Geometry check sheet. Reference: the model listing, model coordinates, mm. Coordinates: 2 decimals unless noted, no trailing zeros. Write each loop counter-clockwise with the first axis right and the second up, starting at its lowest first coordinate (ties: lowest second). Pieces come first, ordered by that corner, then holes. Notation, with made-up numbers: (54.25, 28.5) -> (68.25, 28.5) arc R21 cw to (68.25, 51.5) -> close; hole circle Ø6 at (-14.5, 27.5). An arc over 180 degrees is marked (long way). One line per question, with ' | ' between items.
```python
from build123d import *

# Parameters (mm, degrees)
F1_DEPTH = 6.8
F2_SIZE  = 2.54
F3_SIZE  = 0.508
F5_DEPTH = 6.801


with BuildPart() as f1:
    # F0 (on Top) → F1 (new body)
    with BuildSketch(Plane.XY):
        with BuildLine():
            ThreePointArc((0, -11.175), (-7.9019182798, -7.9019182798), (-11.175, 0))
            Line((-11.175, 0), (-19.135426009, 0))
            ThreePointArc((-19.135426009, 0), (-13.5307894918, -13.5307894918), (0, -19.135426009))
            Line((0, -19.135426009), (0, -11.175))
        make_face()
        with BuildLine():
            Line((-19.135426009, 0), (-11.175, 0))
            ThreePointArc((-11.175, 0), (-10.3243537758, 4.2764873567), (-7.9019182798, 7.9019182798))
            Line((-7.9019182798, 7.9019182798), (-10.1350344611, 10.1350344611))
            ThreePointArc((-10.1350344611, 10.1350344611), (-13.6801442317, 7.7438710244), (-17.8637937449, 6.8592566349))
            ThreePointArc((-17.8637937449, 6.8592566349), (-18.8148323403, 3.4880671653), (-19.135426009, 0))
        make_face()
        with BuildLine():
            ThreePointArc((-7.9019182798, 7.9019182798), (-4.2764873567, 10.3243537758), (0, 11.175))
            Line((0, 11.175), (0, 19.135426009))
            ThreePointArc((0, 19.135426009), (-3.4923449173, 18.8140387882), (-6.8673791432, 17.8606727826))
            ThreePointArc((-6.8673791432, 17.8606727826), (-7.7488210815, 13.6796226746), (-10.1350344611, 10.1350344611))
            Line((-10.1350344611, 10.1350344611), (-7.9019182798, 7.9019182798))
        make_face()
        with BuildLine():
            Line((0, 19.135426009), (0, 11.175))
            ThreePointArc((0, 11.175), (7.9019182798, 7.9019182798), (11.175, 0))
            Line((11.175, 0), (19.135426009, 0))
            ThreePointArc((19.135426009, 0), (13.5307894918, 13.5307894918), (0, 19.135426009))
        make_face()
        with BuildLine():
            Line((19.135426009, 0), (11.175, 0))
            ThreePointArc((11.175, 0), (10.3243537758, -4.2764873567), (7.9019182798, -7.9019182798))
            Line((7.9019182798, -7.9019182798), (10.139134376, -10.139134376))
            ThreePointArc((10.139134376, -10.139134376), (13.6813541851, -7.7515602366), (17.8606227185, -6.8675093486))
            ThreePointArc((17.8606227185, -6.8675093486), (18.8140260583, -3.4924134951), (19.135426009, 0))
        make_face()
        with BuildLine():
            ThreePointArc((7.9019182798, -7.9019182798), (4.2764873567, -10.3243537758), (0, -11.175))
            Line((0, -11.175), (0, -19.135426009))
            ThreePointArc((0, -19.135426009), (3.4924134951, -18.8140260583), (6.8675093486, -17.8606227185))
            ThreePointArc((6.8675093486, -17.8606227185), (7.7515602366, -13.6813541851), (10.139134376, -10.139134376))
            Line((10.139134376, -10.139134376), (7.9019182798, -7.9019182798))
        make_face()
        with BuildLine():
            Line((-36.0821053116, 0), (-19.135426009, 0))
            ThreePointArc((-19.135426009, 0), (-18.8148323403, 3.4880671653), (-17.8637937449, 6.8592566349))
            ThreePointArc((-17.8637937449, 6.8592566349), (-22.2382076575, 7.6759923472), (-25.9470708504, 10.1350344611))
            Line((-25.9470708504, 10.1350344611), (-36.0821053116, 0))
        make_face()
        with BuildLine():
            ThreePointArc((-6.8673791432, 17.8606727826), (-3.4923449173, 18.8140387882), (0, 19.135426009))
            Line((0, 19.135426009), (0, 36.0821053116))
            Line((0, 36.0821053116), (-10.1432364193, 25.9388688923))
            ThreePointArc((-10.1432364193, 25.9388688923), (-7.7178089445, 22.3120170041), (-6.8660526558, 18.0328506976))
            ThreePointArc((-6.8660526558, 18.0328506976), (-6.8663842826, 17.9467591853), (-6.8673791432, 17.8606727826))
        make_face()
        with BuildLine():
            Line((36.0821053116, 0), (19.135426009, 0))
            ThreePointArc((19.135426009, 0), (18.8140260583, -3.4924134951), (17.8606227185, -6.8675093486))
            ThreePointArc((17.8606227185, -6.8675093486), (22.2340501678, -7.6825104386), (25.9429709355, -10.139134376))
            Line((25.9429709355, -10.139134376), (36.0821053116, 0))
        make_face()
        with BuildLine():
            ThreePointArc((6.8675093486, -17.8606227185), (3.4924134951, -18.8140260583), (0, -19.135426009))
            Line((0, -19.135426009), (0, -36.0821053116))
            Line((0, -36.0821053116), (10.139134376, -25.9429709355))
            ThreePointArc((10.139134376, -25.9429709355), (7.6825104386, -22.2340501678), (6.8675093486, -17.8606227185))
        make_face()
        with BuildLine():
            Line((-36.0821053116, 36.0821053116), (-36.0821053116, 0))
            Line((-36.0821053116, 0), (-25.9470708504, 10.1350344611))
            ThreePointArc((-25.9470708504, 10.1350344611), (-29.2160511508, 18.0386503579), (-25.9388688923, 25.9388688923))
            Line((-25.9388688923, 25.9388688923), (-36.0821053116, 36.0821053116))
        make_face()
        with BuildLine():
            Line((-10.1432364193, 25.9388688923), (0, 36.0821053116))
            Line((0, 36.0821053116), (-36.0821053116, 36.0821053116))
            Line((-36.0821053116, 36.0821053116), (-25.9388688923, 25.9388688923))
            ThreePointArc((-25.9388688923, 25.9388688923), (-18.0410526558, 29.2078506976), (-10.1432364193, 25.9388688923))
        make_face()
        with BuildLine():
            Line((36.0821053116, -36.0821053116), (36.0821053116, 0))
            Line((36.0821053116, 0), (25.9429709355, -10.139134376))
            ThreePointArc((25.9429709355, -10.139134376), (28.3654064316, -13.7645652991), (29.2160526558, -18.0410526558))
            ThreePointArc((29.2160526558, -18.0410526558), (28.3654064316, -22.3175400125), (25.9429709355, -25.9429709355))
            Line((25.9429709355, -25.9429709355), (36.0821053116, -36.0821053116))
        make_face()
        with BuildLine():
            Line((10.139134376, -25.9429709355), (0, -36.0821053116))
            Line((0, -36.0821053116), (36.0821053116, -36.0821053116))
            Line((36.0821053116, -36.0821053116), (25.9429709355, -25.9429709355))
            ThreePointArc((25.9429709355, -25.9429709355), (18.0410526558, -29.2160526558), (10.139134376, -25.9429709355))
        make_face()
    extrude(amount=F1_DEPTH)

    # F2
    f2_edges = [f1.edges().sort_by_distance(p)[0] for p in [
        (-13.530789, -13.530789, 6.8),
        (-13.530789, -13.530789, 0),
        (-27.608766, 0, 6.8),
        (-27.608766, 0, 0),
        (18.041053, -36.082105, 6.8),
        (18.041053, -36.082105, 0),
        (0, -27.608766, 0),
        (0, -27.608766, 6.8),
        (36.082105, -18.041053, 6.8),
        (36.082105, -18.041053, 0),
        (27.608766, 0, 0),
        (27.608766, 0, 6.8),
        (13.530789, 13.530789, 6.8),
        (13.530789, 13.530789, 0),
        (0, 27.608766, 6.8),
        (0, 27.608766, 0),
        (-18.041053, 36.082105, 0),
        (-18.041053, 36.082105, 6.8),
        (-36.082105, 18.041053, 6.8),
        (-36.082105, 18.041053, 0),
    ]]
    chamfer(f2_edges, length=F2_SIZE)

    # F3
    f3_edges = [f1.edges().sort_by_distance(p)[0] for p in [
        (-33.542105, 18.041053, 6.8),
        (-24.971, 2.54, 6.8),
        (-11.734738, -11.734738, 6.8),
        (2.54, -24.971, 6.8),
        (18.041053, -33.542105, 6.8),
        (33.542105, -18.041053, 6.8),
        (24.971, -2.54, 6.8),
        (11.734738, 11.734738, 6.8),
        (-2.54, 24.971, 6.8),
        (-18.041053, 33.542105, 6.8),
        (33.542105, -18.041053, 0),
        (18.041053, -33.542105, 0),
        (2.54, -24.971, 0),
        (-11.734738, -11.734738, 0),
        (-24.971, 2.54, 0),
        (-33.542105, 18.041053, 0),
        (-18.041053, 33.542105, 0),
        (-2.54, 24.971, 0),
        (11.734738, 11.734738, 0),
        (24.971, -2.54, 0),
    ]]
    chamfer(f3_edges, length=F3_SIZE)

    # F4 (on face) → F5 (cut, through all)
    with BuildSketch(Plane.XY.offset(6.8)):
        with BuildLine():
            Line((-36.1747518182, 36.0786728561), (-28.1747518182, 36.0786728561))
            ThreePointArc((-28.1747518182, 36.0786728561), (-41.8316060677, 41.7355271056), (-36.1747518182, 28.0786728561))
            Line((-36.1747518182, 28.0786728561), (-36.1747518182, 36.0786728561))
        make_face()
        with BuildLine():
            Line((-28.7767379991, 33.0341053116), (-33.0341053116, 33.0341053116))
            Line((-33.0341053116, 33.0341053116), (-33.0341053116, 28.7209327465))
            ThreePointArc((-33.0341053116, 28.7209327465), (-30.4811848555, 30.4587711451), (-28.7767379991, 33.0341053116))
        make_face()
        with BuildLine():
            Line((-33.0341053116, 28.7209327465), (-33.0341053116, 33.0341053116))
            Line((-33.0341053116, 33.0341053116), (-28.7767379991, 33.0341053116))
            ThreePointArc((-28.7767379991, 33.0341053116), (-28.3266912121, 34.5269174875), (-28.1747518182, 36.0786728561))
            Line((-28.1747518182, 36.0786728561), (-36.1747518182, 36.0786728561))
            Line((-36.1747518182, 36.0786728561), (-36.1747518182, 28.0786728561))
            ThreePointArc((-36.1747518182, 28.0786728561), (-34.5719294445, 28.2408823231), (-33.0341053116, 28.7209327465))
        make_face()
        with BuildLine():
            Line((36.1097641289, -36.1202992499), (36.1097641289, -28.1202992499))
            ThreePointArc((36.1097641289, -28.1202992499), (34.5415065384, -28.2755195761), (33.0341053116, -28.7351572175))
            Line((33.0341053116, -28.7351572175), (33.0341053116, -33.0341053116))
            Line((33.0341053116, -33.0341053116), (28.7290184366, -33.0341053116))
            ThreePointArc((28.7290184366, -33.0341053116), (28.2661053673, -34.5464449902), (28.1097641289, -36.1202992499))
            Line((28.1097641289, -36.1202992499), (36.1097641289, -36.1202992499))
        make_face()
        with BuildLine():
            ThreePointArc((44.1097641289, -36.1202992499), (41.7666183784, -30.4634450004), (36.1097641289, -28.1202992499))
            Line((36.1097641289, -28.1202992499), (36.1097641289, -36.1202992499))
            Line((36.1097641289, -36.1202992499), (28.1097641289, -36.1202992499))
            ThreePointArc((28.1097641289, -36.1202992499), (36.1097641289, -44.1202992499), (44.1097641289, -36.1202992499))
        make_face()
        with BuildLine():
            Line((33.0341053116, -33.0341053116), (33.0341053116, -28.7351572175))
            ThreePointArc((33.0341053116, -28.7351572175), (30.4569473535, -30.459410406), (28.7290184366, -33.0341053116))
            Line((28.7290184366, -33.0341053116), (33.0341053116, -33.0341053116))
        make_face()
    extrude(amount=-F5_DEPTH, mode=Mode.SUBTRACT)


solid = f1.part
```
(1) Depth check by flat-ended pin: P1, Ø4, axis at y = 14, z = 5.5, coming from the +X side; P2, Ø1.4, axis at x = 27, z = 3.5, coming from the +Y side; P3, Ø4, axis at x = -22.5, z = 2, coming from the -Y side. Enter the tip coordinate at first touch or a pass-through.
Answers below:
P1: stops at x = 14.55 | P2: stops at y = 0 | P3: stops at y = 0
(2) Cross-section at A-A (y = -21.5). Record the cut outline in (x, z).
Answers below:
outline: (0, 2.54) -> (2.18, 0.36) -> (3.05, 0) -> (7.41, 0) -> (7.41, 6.8) -> (3.05, 6.8) -> (2.18, 6.44) -> (0, 4.26) -> close; (28.67, 0) -> (33.03, 0) -> (33.9, 0.36) -> (36.08, 2.54) -> (36.08, 4.26) -> (33.9, 6.44) -> (33.03, 6.8) -> (28.67, 6.8) -> close
(3) Cross-section at B-B (z = 1.25). Count the separate pieces of the cut face and the enclosed holes in it, plus the area to 3 significant figures.
Answers below:
separate pieces: 1 | enclosed holes: 3 | area: 1,590 mm²
(4) Material ranges on line 1 (Y direction, x = 10, z = 5.5); line 2 (X direction, y = -8.5, z = 1.5); line 3 (X direction, y = 23.5, z = 6.25), recorded low to high.
Answers below:
line 1: y = -34.84 to -25.8, -10.28 to -4.99, 4.99 to 14.84 | line 2: x = -15.97 to -7.25, 7.25 to 12.22, 23.86 to 35.04 | line 3: x = -34.09 to -27.79, -8.29 to -1.99
